from build123d import *

# Parameters (mm, degrees)
SKETCH1_W                   = 53.975
SKETCH1_H                   = 47.625
BASE_FLANGE1_DEPTH          = 9.525
F_1_4_20_TAPPED_HOLE1_D     = 5.1054
F_1_4_20_TAPPED_HOLE1_DEPTH = 19.05
F_1_4_20_TAPPED_HOLE1_TIP   = 1.533816902
CUT_EXTRUDE1_DEPTH          = 38.230175094
CUT_EXTRUDE2_REACH          = 39.23
F_1_4_20_TAPPED_HOLE2_D     = 5.1054
F_1_4_20_TAPPED_HOLE2_DEPTH = 9.525
CUT_EXTRUDE3_REACH          = 39.23
FILLET2_R                   = 1.5875
FILLET1_R                   = 9.525


# Sheet-metal steps are written as plain solids
with BuildPart() as part:
    # Sketch1 → Base-Flange1 (new body)
    with BuildSketch(Plane.XY):
        Rectangle(SKETCH1_W, SKETCH1_H)
    extrude(amount=BASE_FLANGE1_DEPTH)

    # 1/4-20 Tapped Hole1
    with Locations(Plane(origin=(0, 23.8125, 0), x_dir=(1, 0, 0), z_dir=(0, 1, 0))):
        with Locations((-3.175, -4.7625), (19.05, -4.7625)):
            Hole(F_1_4_20_TAPPED_HOLE1_D / 2, depth=F_1_4_20_TAPPED_HOLE1_DEPTH)
            with Locations((0, 0, -(F_1_4_20_TAPPED_HOLE1_DEPTH + F_1_4_20_TAPPED_HOLE1_TIP / 2))):  # 118° drill point
                Cone(0, F_1_4_20_TAPPED_HOLE1_D / 2, F_1_4_20_TAPPED_HOLE1_TIP, mode=Mode.SUBTRACT)

    # Sketch4 → Cut-Extrude1 (cut, through all)
    with BuildSketch(Plane(origin=(0, 0, 0), x_dir=(-1, 0, 0), z_dir=(0, 0, -1))):
        with BuildLine():
            Line((17.5895, -14.224), (17.5895, -14.351))
            ThreePointArc((17.5895, -14.351), (17.4625, -14.478), (17.3355, -14.351))
            Line((17.3355, -14.351), (17.3355, -14.224))
            ThreePointArc((17.3355, -14.224), (17.4625, -14.097), (17.5895, -14.224))
        make_face()
    extrude(amount=-CUT_EXTRUDE1_DEPTH, mode=Mode.SUBTRACT)

    # Sketch5 → Cut-Extrude2 (cut, up to next)
    with BuildSketch(Plane.XY.offset(9.525), mode=Mode.PRIVATE) as cut_extrude2_sk1:
        Polygon((26.9875, -23.8125), (26.9875, 7.9375), (-7.9375, -23.8125), align=None)
    cut_extrude2_tool1 = extrude(cut_extrude2_sk1.sketch, amount=-CUT_EXTRUDE2_REACH, mode=Mode.PRIVATE) & part.part
    add(cut_extrude2_tool1.solids().sort_by_distance((15.345833, -13.229167, 9.525))[0], mode=Mode.SUBTRACT)

    # 1/4-20 Tapped Hole2
    with Locations(Plane.XY.offset(9.525)):
        with Locations((-17.4625, -14.2875)):
            Hole(F_1_4_20_TAPPED_HOLE2_D / 2, depth=F_1_4_20_TAPPED_HOLE2_DEPTH)

    # Sketch8 → Cut-Extrude3 (cut, up to next)
    with BuildSketch(Plane.XY.offset(9.525), mode=Mode.PRIVATE) as cut_extrude3_sk1:
        Polygon((-26.9875, -4.7625), (-11.1125, 7.9375), (-11.1125, 23.8125), (-26.9875, 23.8125), align=None)
    cut_extrude3_tool1 = extrude(cut_extrude3_sk1.sketch, amount=-CUT_EXTRUDE3_REACH, mode=Mode.PRIVATE) & part.part
    add(cut_extrude3_tool1.solids().sort_by_distance((-19.805952, 12.397619, 9.525))[0], mode=Mode.SUBTRACT)

    # Fillet2
    fillet2_edges = [part.edges().sort_by_distance(p)[0] for p in [
        (-11.1125, 23.8125, 4.7625),
        (26.9875, 23.8125, 4.7625),
    ]]
    fillet(fillet2_edges, radius=FILLET2_R)

    # Fillet1
    fillet1_edges = [part.edges().sort_by_distance(p)[0] for p in [
        (-7.9375, -23.8125, 4.7625),
        (26.9875, 7.9375, 4.7625),
        (-11.1125, 7.9375, 4.7625),
        (-26.9875, -4.7625, 4.7625),
        (-26.9875, -23.8125, 4.7625),
    ]]
    fillet(fillet1_edges, radius=FILLET1_R)


solid = part.part
Build history of the part. All positions in model axes, mm. A direction names the side the tool comes from. Coordinates: 2 decimals unless noted, no trailing zeros. Order: outer loops, then holes, each group sorted by start corner. A loop starts at its lowest first (then second) coordinate and runs counter-clockwise, first axis right, second up. Notation, with made-up numbers: (-5.75, -29) - (25.25, -29) arc R30 cw to (25.25, 6) - close; hole circle Ø5 at (-12.5, -38.75). An arc over 180 degrees is marked (long way). Write item = value, one per line. Start each with the question number.
1) Two-plate mould, pull along Y, no slides. Class faces 1 (the face through (16.69, 14.15, 5.74)), 2 (the face through (-26.02, -5.16, 4.7)), 3 (the face through (-15.437, -15.841, 4.696)): pulls with the +Y half, pulls with the -Y half, needs draft (parallel to the pull), parting line crosses it, or undercut.
2) Saw through at C-C on x = -18.5. Write the cut outline in (y, z) (1 decimal), then the cut area to 3 significant figures.
3) Saw through at B-B on y = 21. Count the separate pieces of the cut face and the enclosed holes in it, then the cut area to 3 significant figures.
4) 3-axis set-ups, long thin cutter, end or side, ignore diameter. For faces 4 (the face through (0, 0, 0)), 5 (the face through (-1.29, 14.15, 3.04)): which of +Z, -Z, +X, -X, +Y, -Y reach the whole face in a straight line?
5) Wall check: line 1 along X through (y, z) = (22, 3.5); line 2 along Y through (x, z) = (-17.5, 8.75); line 3 along Y through (x, z) = (24, 5). Give the ranges that are in metal, low to high. Write a range as from..to.
6) Saw through at D-D on y = -13. Write the cut outline in (x, z) (1 decimal), then the cut area to 3 significant figures.
7) Flat gauge pins, fed straight in: pin 1 Ø1.5 at (y, z) = (10, 3) entering from -X; pin 2 Ø3 at (x, z) = (19.05, 4.76) entering from +Y; pin 3 Ø1.5 at (x, z) = (-3, 1) entering from -Y. Where does each tip first touch, or does it go through?
From the geometry:
q1.face_1 = needs draft
q1.face_2 = pulls with the +Y half
q1.face_3 = undercut
q2.outline = (-23.8, 0) - (-16.6, 0) - (-16.6, 9.5) - (-23.8, 9.5) - close; (-12, 0) - (2, 0) - (2, 9.5) - (-12, 9.5) - close
q2.area = 201 mm^2
q3.separate_pieces = 1
q3.enclosed_holes = 2
q3.area = 322 mm^2
q4.face_4 = -Z, +X, -X, +Y, -Y
q4.face_5 = +Y
q5.line_1 = -11.11..-5.39, -0.96..16.83, 21.27..26.99
q5.line_2 = -23.81..-16.84, -11.74..2.83
q5.line_3 = 5.22..23.81
q6.outline = (-27, 0) - (-19.7, 0) - (-19.7, 9.5) - (-27, 9.5) - close; (-15.3, 0) - (4, 0) - (4, 9.5) - (-15.3, 9.5) - close
q6.area = 253 mm^2
q7.pin_1 = -11.69
q7.pin_2 = 4.13
q7.pin_3 = -20.01
